Input: part model. Units: mm. Frame: model coordinates. Face numbers are marked on the shaded views. Round coordinates to 2 decimals unless told otherwise and drop trailing zeros. Loops run counter-clockwise (first coordinate to the right, second up) from the corner with the lowest first, then second, coordinate; pieces in that order, holes last.
1) Section D-D, the plane x = 25.5. Return loops of the section in (y, z), and give its area (3 significant figures).
2) Ray query, line 1 along X through (y, z) = (7.5, -23); line 2 along X through (y, z) = (5, -21). Return the intervals inside material, ascending.
3) Section C-C, the plane y = 2. Return loops of the section in (x, z).
4) Section B-B, the plane z = -23. Return loops of the section in (x, y).
5) First-contact query: pin 1 (3 mm diameter, centred on x = 27, z = -23, fed in from -Y). Flat tip, straight axial feed; report the tip coordinate or a pass-through.
6) Section A-A, the plane x = 7. Return loops of the section in (y, z), and give its area (3 significant figures).
7) Draft query along X for the marked faces 1, 2 and 3. Return one class per face: pulls with the +X half, pulls with the -X half, needs draft (parallel to the pull), parting line crosses it, or undercut.
from build123d import *

# Parameters (mm, degrees)
SKETCH2_W           = 34
SKETCH2_H           = 33
BOSS_EXTRUDE1_DEPTH = 10
FILLET1_R           = 2
FILLET2_R           = 2
FILLET3_R           = 2
FILLET4_R           = 2
SKETCH3_R           = 2.5
CUT_EXTRUDE1_DEPTH  = 10


with BuildPart() as part:
    # Sketch2 → Boss-Extrude1 (new body)
    with BuildSketch(Plane(origin=(0, 0, 0), x_dir=(1, 0, 0), z_dir=(0, 1, 0))):
        with Locations((17, 16.5)):
            Rectangle(SKETCH2_W, SKETCH2_H)
    extrude(amount=BOSS_EXTRUDE1_DEPTH)

    # Fillet1
    fillet1_edges = [part.edges().sort_by_distance(p)[0] for p in [
        (34, 5, 0),
    ]]
    fillet(fillet1_edges, radius=FILLET1_R)

    # Fillet2
    fillet2_edges = [part.edges().sort_by_distance(p)[0] for p in [
        (34, 5, -33),
    ]]
    fillet(fillet2_edges, radius=FILLET2_R)

    # Fillet3
    fillet3_edges = [part.edges().sort_by_distance(p)[0] for p in [
        (0, 5, -33),
    ]]
    fillet(fillet3_edges, radius=FILLET3_R)

    # Fillet4
    fillet4_edges = [part.edges().sort_by_distance(p)[0] for p in [
        (0, 5, 0),
    ]]
    fillet(fillet4_edges, radius=FILLET4_R)

    # Sketch3 → Cut-Extrude1 (cut)
    with BuildSketch(Plane(origin=(0, 10, 0), x_dir=(1, 0, 0), z_dir=(0, 1, 0))):
        with Locations(Location((7, 23, 0), (0, 0, 270))):
            Circle(SKETCH3_R)
        with Locations(Location((27, 23, 0), (0, 0, 270))):
            Circle(SKETCH3_R)
    extrude(amount=-CUT_EXTRUDE1_DEPTH, mode=Mode.SUBTRACT)


solid = part.part
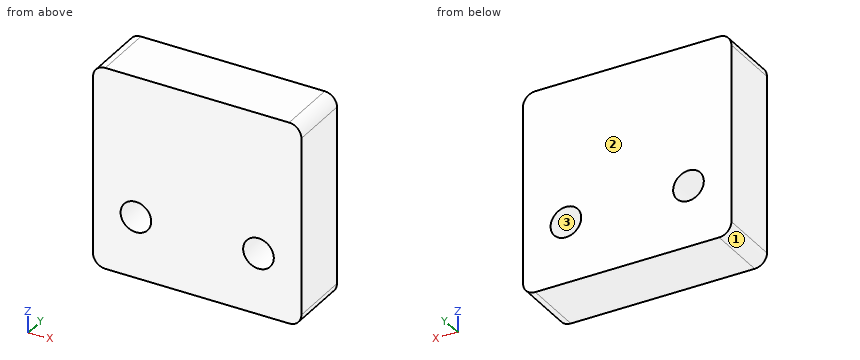
Final values:
1. outline: (0, -33) - (10, -33) - (10, -25) - (0, -25) - close; (0, -21) - (10, -21) - (10, 0) - (0, 0) - close
1. area: 290 mm2
2. line 1: x = 0 to 4.5, 9.5 to 24.5, 29.5 to 34
2. line 2: x = 0 to 5.5, 8.5 to 25.5, 28.5 to 34
3. outline: (0, -31) arc R2 ccw to (2, -33) - (32, -33) arc R2 ccw to (34, -31) - (34, -2) arc R2 ccw to (32, 0) - (2, 0) arc R2 ccw to (0, -2) - close; hole circle Ø5 at (7, -23); hole circle Ø5 at (27, -23)
4. outline: (0, 0) - (4.5, 0) - (4.5, 10) - (0, 10) - close; (9.5, 0) - (24.5, 0) - (24.5, 10) - (9.5, 10) - close; (29.5, 0) - (34, 0) - (34, 10) - (29.5, 10) - close
5. pin 1: passes through
6. outline: (0, -33) - (10, -33) - (10, -25.5) - (0, -25.5) - close; (0, -20.5) - (10, -20.5) - (10, 0) - (0, 0) - close
6. area: 280 mm2
7. face 1: pulls with the -X half
7. face 2: needs draft
7. face 3: undercut
